Geometry check sheet. Reference: the model listing, model coordinates, mm. Face numbers are marked on the shaded views. A direction names the side the tool comes from. Give positions to 0.01 mm unless a question says otherwise; leave off trailing zeros. Write each loop counter-clockwise with the first axis right and the second up, starting at its lowest first coordinate (ties: lowest second). Pieces come first, ordered by that corner, then holes. Notation, with made-up numbers: (-4.5, -17.5) -> (7.5, -17.5) arc R3 ccw to (7.5, -13.5) -> close; hole circle Ø10 at (72, 45). An arc over 180 degrees is marked (long way). One line per item, written item: value.
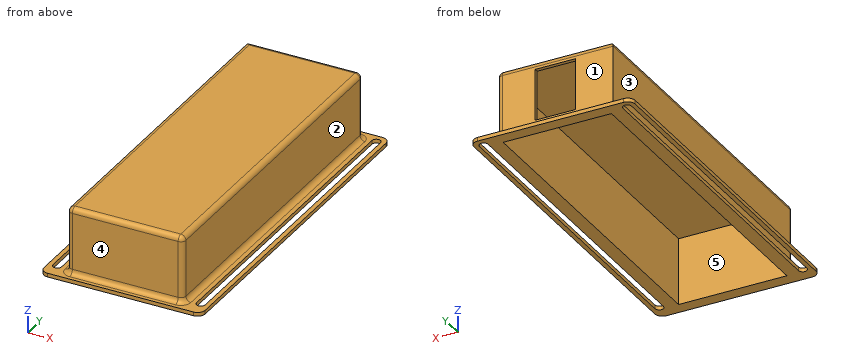
from build123d import *

# Parameters (mm, degrees)
BOSS_EXTRUDE1_DEPTH = 1.5
SKETCH2_W           = 46
SKETCH2_H           = 133
BOSS_EXTRUDE2_DEPTH = 26.5
SKETCH3_W           = 43
SKETCH3_H           = 130
CUT_EXTRUDE1_DEPTH  = 26.5
CUT_EXTRUDE2_DEPTH  = 1.5
SKETCH5_W           = 16
SKETCH5_H           = 20.5
CUT_EXTRUDE3_DEPTH  = 1.5
FILLET1_R           = 2


with BuildPart() as part:
    # Sketch1 → Boss-Extrude1 (new body)
    with BuildSketch(Plane.XY):
        with BuildLine():
            Line((-29, 70), (29, 70))
            ThreePointArc((29, 70), (31.121320344, 69.121320344), (32, 67))
            Line((32, 67), (32, -67))
            ThreePointArc((32, -67), (31.121320344, -69.121320344), (29, -70))
            Line((29, -70), (-29, -70))
            ThreePointArc((-29, -70), (-31.121320344, -69.121320344), (-32, -67))
            Line((-32, -67), (-32, 67))
            ThreePointArc((-32, 67), (-31.121320344, 69.121320344), (-29, 70))
        make_face()
    extrude(amount=BOSS_EXTRUDE1_DEPTH)

    # Sketch2 → Boss-Extrude2 (add)
    with BuildSketch(Plane.XY.offset(1.5)):
        Rectangle(SKETCH2_W, SKETCH2_H)
    extrude(amount=BOSS_EXTRUDE2_DEPTH)

    # Sketch3 → Cut-Extrude1 (cut)
    with BuildSketch(Plane(origin=(0, 0, 0), x_dir=(-1, 0, 0), z_dir=(0, 0, -1))):
        Rectangle(SKETCH3_W, SKETCH3_H)
    extrude(amount=-CUT_EXTRUDE1_DEPTH, mode=Mode.SUBTRACT)

    # Sketch4 → Cut-Extrude2 (cut)
    with BuildSketch(Plane(origin=(0, 0, 0), x_dir=(-1, 0, 0), z_dir=(0, 0, -1))):
        with BuildLine():
            Line((-30.2, 66.330000504), (-30.2, -63.669999496))
            ThreePointArc((-30.2, -63.669999496), (-28.5, -65.369999496), (-26.8, -63.669999496))
            Line((-26.8, -63.669999496), (-26.8, 66.330000504))
            ThreePointArc((-26.8, 66.330000504), (-28.5, 68.030000504), (-30.2, 66.330000504))
        make_face()
        with BuildLine():
            Line((30.2, 66.330000504), (30.2, -63.669999496))
            ThreePointArc((30.2, -63.669999496), (28.5, -65.369999496), (26.8, -63.669999496))
            Line((26.8, -63.669999496), (26.8, 66.330000504))
            ThreePointArc((26.8, 66.330000504), (28.5, 68.030000504), (30.2, 66.330000504))
        make_face()
    extrude(amount=-CUT_EXTRUDE2_DEPTH, mode=Mode.SUBTRACT)

    # Sketch5 → Cut-Extrude3 (cut)
    with BuildSketch(Plane(origin=(0, 66.5, 0), x_dir=(1, 0, 0), z_dir=(0, 1, 0))):
        with Locations((0, -14.75)):
            Rectangle(SKETCH5_W, SKETCH5_H)
    extrude(amount=-CUT_EXTRUDE3_DEPTH, mode=Mode.SUBTRACT)

    # Fillet1
    fillet1_edges = [part.edges().sort_by_distance(p)[0] for p in [
        (23, 0, 1.5),
        (23, -66.5, 14.75),
        (0, 66.5, 1.5),
        (23, 66.5, 14.75),
        (-23, 0, 1.5),
        (0, -66.5, 1.5),
        (-23, -66.5, 14.75),
        (23, 0, 28),
        (0, 66.5, 28),
        (-23, 0, 28),
        (0, -66.5, 28),
    ]]
    fillet(fillet1_edges, radius=FILLET1_R)


solid = part.part
1) Sectioned sample at C-C on z = 18.75. Record the cut outline in (x, y), plus the area to 3 significant figures.
Verdict:
outline: (-23, -64.5) arc R2 ccw to (-21, -66.5) -> (21, -66.5) arc R2 ccw to (23, -64.5) -> (23, 64.5) arc R2 ccw to (21, 66.5) -> (8, 66.5) -> (8, 65) -> (21.5, 65) -> (21.5, -65) -> (-21.5, -65) -> (-21.5, 65) -> (-8, 65) -> (-8, 66.5) -> (-23, 66.5) -> close
area: 501 mm^2
2) Tool access check on the marked faces 1, 2, 3, 4 and 5. Record the directions out of +Z, -Z, +X, -X, +Y, -Y that give a thin tool (end or side, any length) a straight path to the whole face; none if there is none.
Verdict:
face 1: +Z, +X, -X, +Y
face 2: +Z, +X, +Y, -Y
face 3: +Z, -X, +Y, -Y
face 4: +Z, +X, -X, -Y
face 5: -Z
3) Scan lines: probe 1 along Y at (x, z) = (-12, 20.75); probe 2 along X at (y, z) = (-46, 24); probe 3 along Z at (x, y) = (-15, 61.5). Record each from-to range of solid material in increasing order.
Verdict:
probe 1: -66.5 to -65, 65 to 66.5
probe 2: -23 to -21.5, 21.5 to 23
probe 3: 26.5 to 28
4) Sectioned sample at D-D on x = 17.5. Record the cut outline in (y, z), plus the area to 4 significant figures.
Verdict:
outline: (-70, 0) -> (-65, 0) -> (-65, 26.5) -> (65, 26.5) -> (65, 0) -> (70, 0) -> (70, 1.5) -> (68.5, 1.5) arc R2 cw to (66.5, 3.5) -> (66.5, 26) arc R2 ccw to (64.5, 28) -> (-64.5, 28) arc R2 ccw to (-66.5, 26) -> (-66.5, 3.5) arc R2 cw to (-68.5, 1.5) -> (-70, 1.5) -> close
area: 289.5 mm^2
5) Sectioned sample at B-B on y = 6.5. Record the cut outline in (x, z).
Verdict:
outline: (-32, 0) -> (-30.2, 0) -> (-30.2, 1.5) -> (-32, 1.5) -> close; (-26.8, 0) -> (-21.5, 0) -> (-21.5, 26.5) -> (21.5, 26.5) -> (21.5, 0) -> (26.8, 0) -> (26.8, 1.5) -> (25, 1.5) arc R2 cw to (23, 3.5) -> (23, 26) arc R2 ccw to (21, 28) -> (-21, 28) arc R2 ccw to (-23, 26) -> (-23, 3.5) arc R2 cw to (-25, 1.5) -> (-26.8, 1.5) -> close; (30.2, 0) -> (32, 0) -> (32, 1.5) -> (30.2, 1.5) -> close
6) Sectioned sample at A-A on x = -0.5. Record the cut outline in (y, z), plus the area to 3 significant figures.
Verdict:
outline: (-70, 0) -> (-65, 0) -> (-65, 26.5) -> (65, 26.5) -> (65, 25) -> (66.5, 25) -> (66.5, 26) arc R2 ccw to (64.5, 28) -> (-64.5, 28) arc R2 ccw to (-66.5, 26) -> (-66.5, 3.5) arc R2 cw to (-68.5, 1.5) -> (-70, 1.5) -> close; (65, 0) -> (70, 0) -> (70, 1.5) -> (68.5, 1.5) arc R2 cw to (66.5, 3.5) -> (66.5, 4.5) -> (65, 4.5) -> close
area: 259 mm^2
7) Depth check by flat-ended pin: pin 1 Ø8 at (y, z) = (-41, 21.5) entering from -X; pin 2 Ø8 at (x, z) = (-2.5, 13) entering from +Y; pin 3 Ø3 at (x, z) = (17.5, 6.5) entering from -Y. Enter the tip coordinate at first touch or a pass-through.
Verdict:
pin 1: x = -23
pin 2: y = -65
pin 3: y = -66.5
